Print and shaded views of the part. All mm, measured from the part's lowest x, y and z. A direction names the side the tool comes from. Give positions to 0.01 mm unless a question says otherwise; leave off trailing zeros. Write each loop counter-clockwise with the first axis right and the second up, starting at its lowest first coordinate (ties: lowest second). Pieces come first, ordered by that corner, then holes. Notation, with made-up numbers: (12.5, 42.5) -> (62.5, 42.5) arc R21 ccw to (62.5, 69.5) -> close; hole circle Ø3 at (43.5, -8.75). An arc over 180 degrees is marked (long way). Put each result on its own line as item: value.
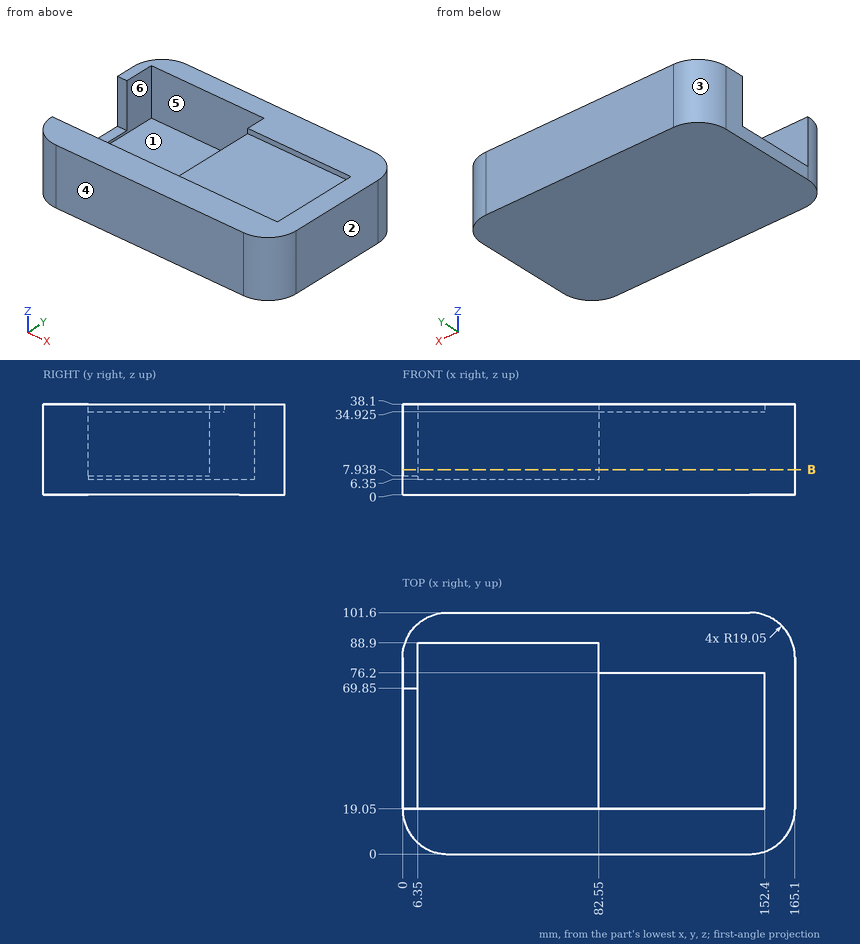
1) Tool access for the marked faces 1 and 2: list every direction of +Z, -Z, +X, -X, +Y, -Y with a clear straight run to the whole face (end or side of a thin tool).
Filled sheet:
face 1: +Z
face 2: +Z, -Z, +X, +Y, -Y
2) Pull direction X, two halves, no side cores. Call the marked faces 3, 4, 5 and 6: released by +X, released by -X, zero draft, split by the parting line, or undercut.
Filled sheet:
face 3: released by -X
face 4: zero draft
face 5: undercut
face 6: undercut
3) Pin check, flat tips, straight feed: pin 1 (16 mm diameter, centred on y = 62, z = 20.5, fed in from -X); pin 2 (17 mm diameter, centred on x = 115.5, y = 57.5, fed in from +Z) (1 decimal); pin 3 (8 mm diameter, centred on x = 69, y = 50, fed in from +Z); pin 4 (5 mm diameter, centred on x = 3, y = 56, fed in from +Z). Stop position of each tip, or through.
Filled sheet:
pin 1: x = 0
pin 2: z = 34.9
pin 3: z = 6.35
pin 4: z = 7.94
4) Slice it at B-B (z = 10.5). Write the cut outline in (x, y).
Filled sheet:
outline: (0, 19.05) arc R19.05 ccw to (19.05, 0) -> (146.05, 0) arc R19.05 ccw to (165.1, 19.05) -> (165.1, 82.55) arc R19.05 ccw to (146.05, 101.6) -> (19.05, 101.6) arc R19.05 ccw to (0, 82.55) -> (0, 69.85) -> (6.35, 69.85) -> (6.35, 88.9) -> (82.55, 88.9) -> (82.55, 19.05) -> close
5) Wall check: L1, parallel to Y at x = 56, z = 34.5; L2, parallel to X at y = 70, z = 27; L3, parallel to Z at x = 134, y = 58.5 (1 decimal). Give the ranges that are in metal, low to high.
Filled sheet:
L1: 0 to 19.05, 88.9 to 101.6
L2: 0 to 6.35, 82.55 to 165.1
L3: 0 to 34.9
